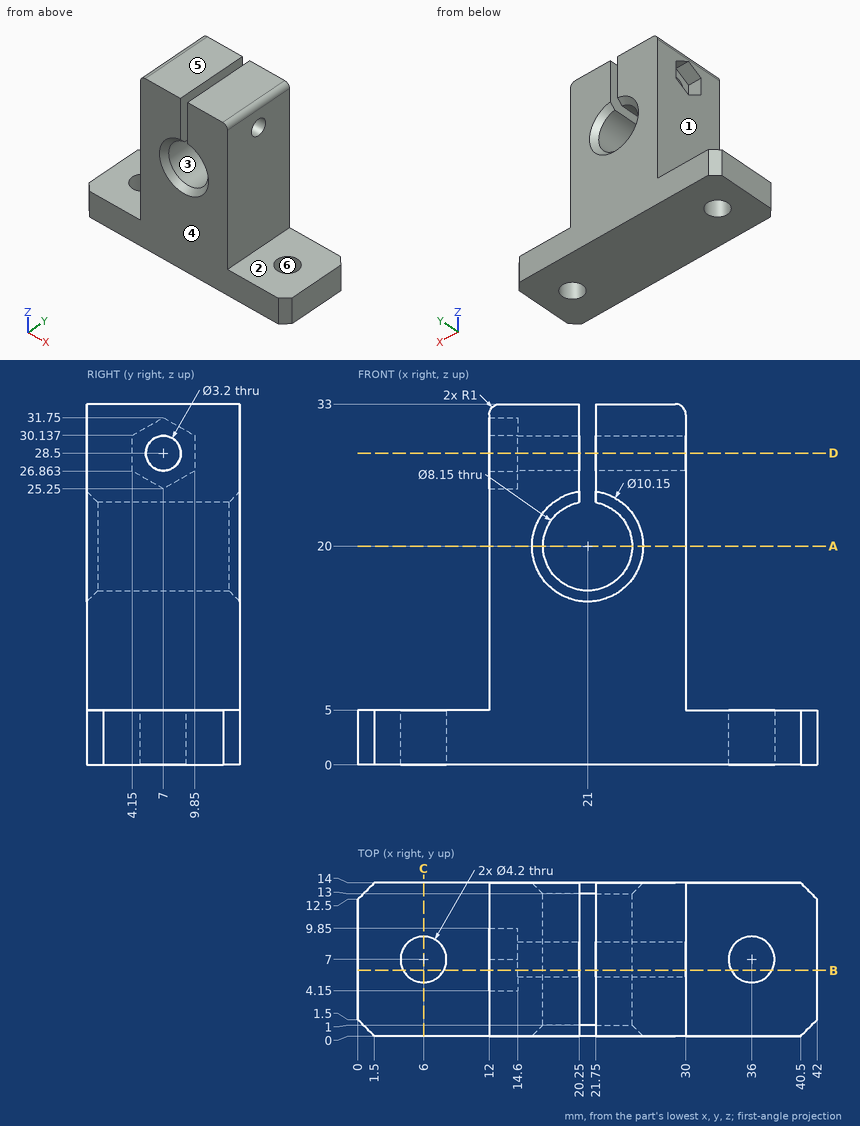
Print and shaded views of the part. All mm, measured from the part's lowest x, y and z. A direction names the side the tool comes from. Give positions to 0.01 mm unless a question says otherwise; leave off trailing zeros. Loops run counter-clockwise (first coordinate to the right, second up) from the corner with the lowest first, then second, coordinate; pieces in that order, holes last.
1) Wall check: line 1 (X direction, y = 13, z = 25); line 2 (Y direction, x = 36, z = 1.9); line 3 (Y direction, x = 16.6, z = 28.5). Give the ranges that are in metal, low to high.
2) Tool access for the marked faces 1, 2 and 3: list every direction of +Z, -Z, +X, -X, +Y, -Y with a clear straight run to the whole face (end or side of a thin tool).
3) Flat gauge pins, fed straight in: pin 1 Ø4 at (y, z) = (3.5, 23) entering from +X; pin 2 Ø2 at (x, z) = (12.5, 21.5) entering from -Y; pin 3 Ø5 at (x, y) = (36, 7) entering from +Z; pin 4 Ø5 at (y, z) = (12.5, 17) entering from -X. Where does each tip first touch, or does it go through?
4) Pull direction Y, two halves, no side cores. Call the marked faces 4, 5 and 6: +Y half, -Y half, draft (parallel to the pull), parting line (faces both ways), or undercut.
5) Saw through at D-D (z = 28.5). Write the cut outline in (x, y).
6) Saw through at A-A (z = 20). Write the cut outline in (x, y) (1 decimal), plus the area to 3 significant figures.
7) Saw through at B-B (y = 6). Count the separate pieces of the cut face and the enclosed holes in it.
8) Saw through at C-C (x = 6). Write the cut outline in (y, z).
Answer block:
1. line 1: x = 12 to 20.25, 21.75 to 30
1. line 2: y = 0 to 4.9, 9.1 to 14
1. line 3: y = 0 to 5.4, 8.6 to 14
2. face 1: +Z, -X, +Y, -Y
2. face 2: +Z, +X, +Y, -Y
2. face 3: +Y, -Y
3. pin 1: stops at x = 30
3. pin 2: stops at y = 0
3. pin 3: stops at z = 5
3. pin 4: stops at x = 12
4. face 4: -Y half
4. face 5: draft
4. face 6: undercut
5. outline: (12, 0) - (20.25, 0) - (20.25, 5.4) - (14.6, 5.4) - (14.6, 4.15) - (12, 4.15) - close; (12, 9.85) - (14.6, 9.85) - (14.6, 8.6) - (20.25, 8.6) - (20.25, 14) - (12, 14) - close; (21.75, 0) - (30, 0) - (30, 5.4) - (21.75, 5.4) - close; (21.75, 8.6) - (30, 8.6) - (30, 14) - (21.75, 14) - close
6. outline: (12, 0) - (15.9, 0) - (16.9, 1) - (16.9, 13) - (15.9, 14) - (12, 14) - close; (25.1, 1) - (26.1, 0) - (30, 0) - (30, 14) - (26.1, 14) - (25.1, 13) - close
6. area: 136 mm2
7. separate pieces: 5
7. enclosed holes: 0
8. outline: (0, 0) - (4.9, 0) - (4.9, 5) - (0, 5) - close; (9.1, 0) - (14, 0) - (14, 5) - (9.1, 5) - close
